```python
from build123d import *

# Parameters (mm, degrees)
F0_W      = 31.75
F0_H      = 31.75
F1_DEPTH  = 60.33
F2_W      = 22.23
F2_H      = 22.23
F3_DEPTH  = 6.35
F4_W      = 31.75
F4_H      = 31.75
F5_DEPTH  = 112.71
F6_W      = 22.23
F6_H      = 22.23
F7_DEPTH  = 6.35
F8_W      = 31.75
F8_H      = 31.75
F8_W_2    = 22.23
F8_H_2    = 22.23
F9_DEPTH  = 112.71
F10_W     = 22.23
F10_H     = 22.23
F11_DEPTH = 6.35
F12_W     = 31.75
F12_H     = 31.75
F12_W_2   = 22.23
F12_H_2   = 22.23
F13_DEPTH = 112.71
F14_W     = 22.23
F14_H     = 22.23
F15_DEPTH = 6.35
F16_W     = 31.75
F16_H     = 31.75
F17_DEPTH = 112.71
F18_W     = 22.23
F18_H     = 22.23
F19_DEPTH = 6.35
F20_W     = 31.75
F20_H     = 31.75
F20_W_2   = 22.23
F20_H_2   = 22.23
F21_DEPTH = 112.71
F22_W     = 22.23
F22_H     = 22.23
F23_DEPTH = 6.35
F24_W     = 31.75
F24_H     = 31.75
F24_W_2   = 22.23
F24_H_2   = 22.23
F25_DEPTH = 25.4
F26_W     = 22.23
F26_H     = 22.23
F27_DEPTH = 6.35
F28_W     = 31.75
F28_H     = 31.75
F28_W_2   = 22.23
F28_H_2   = 22.23
F29_DEPTH = 31.75
F32_DEPTH = 12.7
F34_DEPTH = 12.7
F36_DEPTH = 12.7
F38_DEPTH = 12.7
F40_DEPTH = 12.7
F41_W     = 12.7
F41_H     = 12.7
F42_DEPTH = 736.6
F43_DEPTH = 6.35
F44_W     = 31.75
F44_H     = 360.990007
F45_DEPTH = 76.2
F47_DEPTH = 12.7


with BuildPart() as f1:
    # F0 (on Top) → F1 (new body)
    with BuildSketch(Plane.XY):
        with Locations((15.875, 15.875)):
            Rectangle(F0_W, F0_H)
    extrude(amount=F1_DEPTH)

    # F2 (on face) → F3 (join)
    with BuildSketch(Plane.XY.offset(60.33)):
        with Locations((15.875, 15.875)):
            Rectangle(F2_W, F2_H)
    extrude(amount=F3_DEPTH)

    # F4 (on face) → F5 (join)
    with BuildSketch(Plane.XY.offset(66.68)):
        with Locations((15.875, 15.875)):
            Rectangle(F4_W, F4_H)
    extrude(amount=F5_DEPTH)

    # F6 (on face) → F7 (join)
    with BuildSketch(Plane.XY.offset(179.39)):
        with Locations((15.875, 15.875)):
            Rectangle(F6_W, F6_H)
    extrude(amount=F7_DEPTH)

    # F8 (on face) → F9 (join)
    with BuildSketch(Plane.XY.offset(185.74)):
        with Locations((15.875, 15.875)):
            Rectangle(F8_W, F8_H)
        with Locations((15.875, 15.875)):
            Rectangle(F8_W_2, F8_H_2, mode=Mode.SUBTRACT)
        with Locations((15.875, 15.875)):
            Rectangle(F8_W_2, F8_H_2)
    extrude(amount=F9_DEPTH)

    # F10 (on face) → F11 (join)
    with BuildSketch(Plane.XY.offset(298.45)):
        with Locations((15.875, 15.875)):
            Rectangle(F10_W, F10_H)
    extrude(amount=F11_DEPTH)

    # F12 (on face) → F13 (join)
    with BuildSketch(Plane.XY.offset(304.8)):
        with Locations((15.875, 15.875)):
            Rectangle(F12_W, F12_H)
        with Locations((15.875, 15.875)):
            Rectangle(F12_W_2, F12_H_2, mode=Mode.SUBTRACT)
        with Locations((15.875, 15.875)):
            Rectangle(F12_W_2, F12_H_2)
    extrude(amount=F13_DEPTH)

    # F14 (on face) → F15 (join)
    with BuildSketch(Plane.XY.offset(417.51)):
        with Locations((15.875, 15.875)):
            Rectangle(F14_W, F14_H)
    extrude(amount=F15_DEPTH)

    # F16 (on face) → F17 (join)
    with BuildSketch(Plane.XY.offset(423.86)):
        with Locations((15.875, 15.875)):
            Rectangle(F16_W, F16_H)
    extrude(amount=F17_DEPTH)

    # F18 (on face) → F19 (join)
    with BuildSketch(Plane.XY.offset(536.57)):
        with Locations((15.875, 15.875)):
            Rectangle(F18_W, F18_H)
    extrude(amount=F19_DEPTH)

    # F20 (on face) → F21 (join)
    with BuildSketch(Plane.XY.offset(542.92)):
        with Locations((15.875, 15.875)):
            Rectangle(F20_W, F20_H)
        with Locations((15.875, 15.875)):
            Rectangle(F20_W_2, F20_H_2, mode=Mode.SUBTRACT)
        with Locations((15.875, 15.875)):
            Rectangle(F20_W_2, F20_H_2)
    extrude(amount=F21_DEPTH)

    # F22 (on face) → F23 (join)
    with BuildSketch(Plane.XY.offset(655.63)):
        with Locations((15.875, 15.875)):
            Rectangle(F22_W, F22_H)
    extrude(amount=F23_DEPTH)

    # F24 (on face) → F25 (join)
    with BuildSketch(Plane.XY.offset(661.98)):
        with Locations((15.875, 15.875)):
            Rectangle(F24_W, F24_H)
        with Locations((15.875, 15.875)):
            Rectangle(F24_W_2, F24_H_2, mode=Mode.SUBTRACT)
        with Locations((15.875, 15.875)):
            Rectangle(F24_W_2, F24_H_2)
    extrude(amount=F25_DEPTH)

    # F26 (on face) → F27 (join)
    with BuildSketch(Plane.XY.offset(687.38)):
        with Locations((15.875, 15.875)):
            Rectangle(F26_W, F26_H)
    extrude(amount=F27_DEPTH)

    # F28 (on face) → F29 (join)
    with BuildSketch(Plane.XY.offset(693.73)):
        with Locations((15.875, 15.875)):
            Rectangle(F28_W, F28_H)
        with Locations((15.875, 15.875)):
            Rectangle(F28_W_2, F28_H_2, mode=Mode.SUBTRACT)
        with Locations((15.875, 15.875)):
            Rectangle(F28_W_2, F28_H_2)
    extrude(amount=F29_DEPTH)

    # F31 (on face) → F32 (cut)
    with BuildSketch(Plane.XZ):
        with BuildLine():
            Line((15.875, 123.035), (20.64, 123.035))
            ThreePointArc((20.64, 123.035), (12.5056361876, 126.4043638124), (15.875, 118.27))
            Line((15.875, 118.27), (15.875, 123.035))
        make_face()
        with BuildLine():
            ThreePointArc((15.875, 118.27), (19.2443638124, 119.6656361876), (20.64, 123.035))
            Line((20.64, 123.035), (15.875, 123.035))
            Line((15.875, 123.035), (15.875, 118.27))
        make_face()
    extrude(amount=-F32_DEPTH, mode=Mode.SUBTRACT)

    # F33 (on face) → F34 (cut)
    with BuildSketch(Plane.YZ.offset(31.75)):
        with BuildLine():
            Line((15.875, 242.095), (20.64, 242.095))
            ThreePointArc((20.64, 242.095), (12.5056361876, 245.4643638124), (15.875, 237.33))
            Line((15.875, 237.33), (15.875, 242.095))
        make_face()
        with BuildLine():
            ThreePointArc((15.875, 237.33), (19.2443638124, 238.7256361876), (20.64, 242.095))
            Line((20.64, 242.095), (15.875, 242.095))
            Line((15.875, 242.095), (15.875, 237.33))
        make_face()
    extrude(amount=-F34_DEPTH, mode=Mode.SUBTRACT)

    # F35 (on face) → F36 (cut)
    with BuildSketch(Plane.XZ):
        with BuildLine():
            Line((15.875, 361.155), (20.64, 361.155))
            ThreePointArc((20.64, 361.155), (12.5056361876, 364.5243638124), (15.875, 356.39))
            Line((15.875, 356.39), (15.875, 361.155))
        make_face()
        with BuildLine():
            ThreePointArc((15.875, 356.39), (19.2443638124, 357.7856361876), (20.64, 361.155))
            Line((20.64, 361.155), (15.875, 361.155))
            Line((15.875, 361.155), (15.875, 356.39))
        make_face()
    extrude(amount=-F36_DEPTH, mode=Mode.SUBTRACT)

    # F37 (on face) → F38 (cut)
    with BuildSketch(Plane.YZ.offset(31.75)):
        with BuildLine():
            Line((15.875, 480.215), (20.64, 480.215))
            ThreePointArc((20.64, 480.215), (12.5056361876, 483.5843638124), (15.875, 475.45))
            Line((15.875, 475.45), (15.875, 480.215))
        make_face()
        with BuildLine():
            ThreePointArc((15.875, 475.45), (19.2443638124, 476.8456361876), (20.64, 480.215))
            Line((20.64, 480.215), (15.875, 480.215))
            Line((15.875, 480.215), (15.875, 475.45))
        make_face()
    extrude(amount=-F38_DEPTH, mode=Mode.SUBTRACT)

    # F39 (on face) → F40 (cut)
    with BuildSketch(Plane.XZ):
        with BuildLine():
            Line((15.875, 599.275), (20.64, 599.275))
            ThreePointArc((20.64, 599.275), (12.5056361876, 602.6443638124), (15.875, 594.51))
            Line((15.875, 594.51), (15.875, 599.275))
        make_face()
        with BuildLine():
            ThreePointArc((15.875, 594.51), (19.2443638124, 595.9056361876), (20.64, 599.275))
            Line((20.64, 599.275), (15.875, 599.275))
            Line((15.875, 599.275), (15.875, 594.51))
        make_face()
    extrude(amount=-F40_DEPTH, mode=Mode.SUBTRACT)

    # F41 (on face) → F42 (cut)
    with BuildSketch(Plane.XY.offset(725.48)):
        with Locations((15.87, 15.87)):
            Rectangle(F41_W, F41_H)
    extrude(amount=-F42_DEPTH, mode=Mode.SUBTRACT)

    # F30 (on face) → F43 (cut)
    with BuildSketch(Plane(origin=(0, 0, 0), x_dir=(1, 0, 0), z_dir=(0, 0, -1))):
        with BuildLine():
            ThreePointArc((6.35, -15.875), (9.1398079092, -22.6101920908), (15.875, -25.4))
            Line((15.875, -25.4), (15.875, -15.875))
            Line((15.875, -15.875), (6.35, -15.875))
        make_face()
        with BuildLine():
            Line((15.875, -15.875), (15.875, -25.4))
            ThreePointArc((15.875, -25.4), (22.6101920908, -22.6101920908), (25.4, -15.875))
            ThreePointArc((25.4, -15.875), (15.875, -6.35), (6.35, -15.875))
            Line((6.35, -15.875), (15.875, -15.875))
        make_face()
    extrude(amount=-F43_DEPTH, mode=Mode.SUBTRACT)

    # F44 (on face) → F45 (cut)
    with BuildSketch(Plane.XZ):
        with Locations((15.875, 180.4950035)):
            Rectangle(F44_W, F44_H)
    extrude(amount=-F45_DEPTH, mode=Mode.SUBTRACT)

    # F46 (on face) → F47 (cut)
    with BuildSketch(Plane(origin=(0, 0, 360.990007), x_dir=(1, 0, 0), z_dir=(0, 0, -1))):
        Polygon((11.1128573824, -9.52), (11.1128573824, -3.175), (3.175, -3.175), (3.175, -28.575), (28.575, -28.575), (28.575, -3.175), (20.6371426176, -3.175), (20.6371426176, -9.52), (22.22, -9.52), (22.22, -22.22), (9.52, -22.22), (9.52, -9.52), align=None)
        Polygon((20.6371426176, -3.175), (11.1128573824, -3.175), (11.1128573824, -9.52), (9.52, -9.52), (9.52, -22.22), (22.22, -22.22), (22.22, -9.52), (20.6371426176, -9.52), align=None)
    extrude(amount=-F47_DEPTH, mode=Mode.SUBTRACT)


solid = f1.part
```
Part model, mm, in its own coordinate system. A direction names the side the tool comes from. Round coordinates to 2 decimals unless told otherwise and drop trailing zeros. Write each loop counter-clockwise with the first axis right and the second up, starting at its lowest first coordinate (ties: lowest second). Pieces come first, ordered by that corner, then holes. Notation, with made-up numbers: M -29.75,25.5 L 24.25,25.5 A20 ccw 24.25,62.5 Z; hole C 42.25,-29.75 d1. An arc over 180 degrees is marked long. One line per question, with ' | ' between items.
(1) 3-axis set-ups, long thin cutter, end or side, ignore diameter. For faces 4 (the face through (16, 22.22, 552)), 5 (the face through (28.575, 16, 367)), 6 (the face through (26.99, 16, 659)), 7 (the face through (16, 4.76, 691)), 8 (the face through (16, 2, 423.86)): which of +Z, -Z, +X, -X, +Y, -Y reach the whole face in a straight line?
Answer key:
face 4: +Z, -Z | face 5: -Z | face 6: +X, +Y, -Y | face 7: +X, -X, -Y | face 8: none
(2) Two-plate mould, pull along Z, no slides. Class faces 1 (the face through (26.99, 16, 540)), 2 (the face through (0, 16, 479)), 3 (the face through (4.76, 16, 421)): released by +Z, released by -Z, zero draft, split by the parting line, or undercut.
Answer key:
face 1: undercut | face 2: zero draft | face 3: undercut
(3) Probe line 1 along Z through (x, y) = (29, 24.5); line 2 along Z through (x, y) = (28, 5); line 3 along Y through (x, z) = (14, 627.5). List the from-to ranges inside material, lowest first.
Answer key:
line 1: z = 360.99 to 417.51, 423.86 to 536.57, 542.92 to 655.63, 661.98 to 687.38, 693.73 to 725.48 | line 2: z = 373.69 to 417.51, 423.86 to 536.57, 542.92 to 655.63, 661.98 to 687.38, 693.73 to 725.48 | line 3: y = 0 to 9.52, 22.22 to 31.75
(4) Saw through at A-A on z = 447. Write the cut outline in (x, y).
Answer key:
outline: M 0,0 L 31.75,0 L 31.75,31.75 L 0,31.75 Z; hole M 9.52,9.52 L 22.22,9.52 L 22.22,22.22 L 9.52,22.22 Z
(5) Pin check, flat tips, straight feed: pin 1 (3 mm diameter, centred on x = 26, y = 22.5, fed in from -Z); pin 2 (3 mm diameter, centred on x = 11, z = 540, fed in from -Y); pin 3 (1.9 mm diameter, centred on y = 15, z = 538.5, fed in from -X). Stop position of each tip, or through.
Answer key:
pin 1: stops at z = 373.69 | pin 2: stops at y = 4.76 | pin 3: stops at x = 4.76
